```python
from build123d import *

# Parameters (mm, degrees)
BOSS_EXTRUDE1_DEPTH = 1.5875
FILLET1_R           = 2.54


with BuildPart() as part:
    # Sketch1 → Boss-Extrude1 (new body)
    with BuildSketch(Plane.XY):
        with BuildLine():
            Line((-5.175, 2.670071332), (-5.175, -5.175))
            Line((-5.175, -5.175), (5.175, -5.175))
            Line((5.175, -5.175), (5.175, 2.670071332))
            ThreePointArc((5.175, 2.670071332), (0, 12.7), (-5.175, 2.670071332))
        make_face()
        Polygon((-3.175, -1.5875), (-3.175, 1.5875), (-1.5875, 1.5875), (-1.5875, 3.175), (1.5875, 3.175), (1.5875, 1.5875), (3.175, 1.5875), (3.175, -1.5875), (1.5875, -1.5875), (1.5875, -3.175), (-1.5875, -3.175), (-1.5875, -1.5875), align=None, mode=Mode.SUBTRACT)
    extrude(amount=BOSS_EXTRUDE1_DEPTH)

    # Fillet1
    fillet1_edges = [part.edges().sort_by_distance(p)[0] for p in [
        (5.175, -5.175, 0.79375),
        (-5.175, -5.175, 0.79375),
    ]]
    fillet(fillet1_edges, radius=FILLET1_R)


solid = part.part
```
Input: part model. Units: mm. Frame: model coordinates. A direction names the side the tool comes from. Round coordinates to 2 decimals unless told otherwise and drop trailing zeros. Loops run counter-clockwise (first coordinate to the right, second up) from the corner with the lowest first, then second, coordinate; pieces in that order, holes last. Notation, with made-up numbers: (-2, 35) -> (49, 35) arc R23 ccw to (49, 70) -> close; hole circle Ø2 at (55.5, 84.25). An arc over 180 degrees is marked (long way). One line per item, written item: value.
(1) Section A-A (x = 0). Return the cut outline in (y, z) (1 decimal), plus the area to 3 significant figures.
Geometry check:
outline: (-5.2, 0) -> (-3.2, 0) -> (-3.2, 1.6) -> (-5.2, 1.6) -> close; (3.2, 0) -> (12.7, 0) -> (12.7, 1.6) -> (3.2, 1.6) -> close
area: 18.3 mm2
(2) Pin query (flat end, axial travel): pin 1 (0.5 mm diameter, centred on y = -0.5, z = 1, fed in from -X) (3 decimals); pin 2 (0.8 mm diameter, centred on x = -2, z = 1, fed in from +Y); pin 3 (3 mm diameter, centred on x = -1, y = 6.5, fed in from -Z); pin 4 (0.8 mm diameter, centred on y = 0.5, z = 1, fed in from +X) (3 decimals). Return the tip coordinate at first contact, or that it passes through.
Geometry check:
pin 1: x = -5.175
pin 2: y = 12.5
pin 3: z = 0
pin 4: x = 5.175
(3) Material intervals for line 1 (X direction, y = -0.25, z = 0.4) (3 decimals); line 2 (X direction, y = 2.5, z = 0.4) (1 decimal); line 3 (Y direction, x = -0.75, z = 0.35) (3 decimals), sorted ascending. Write a range as [from, to].
Geometry check:
line 1: [-5.175, -3.175], [3.175, 5.175]
line 2: [-5.2, -1.6], [1.6, 5.2]
line 3: [-5.175, -3.175], [3.175, 12.656]
(4) Set-up query: faces 1 (the face through (-5.175, 0, 1)), 2 (the face through (0, -5.175, 1)), 3 (the face through (0, -3.175, 1)). Return all of +Z, -Z, +X, -X, +Y, -Y with unobstructed straight access to the full face (end or side cutting, diameter ignored); none if empty.
Geometry check:
face 1: +Z, -Z, -X, -Y
face 2: +Z, -Z, +X, -X, -Y
face 3: +Z, -Z
(5) Mould query, pull axis Y, two halves, no side actions, for faces 4 (the face through (2, -1.588, 1)), 5 (the face through (0.195, 12.697, 0.783)), 6 (the face through (5.175, 0, 1)). Classes: pulls with the +Y half, pulls with the -Y half, needs draft (parallel to the pull), parting line crosses it, or undercut.
Geometry check:
face 4: undercut
face 5: parting line crosses it
face 6: needs draft
(6) Section C-C (x = -4). Return the cut outline in (y, z).
Geometry check:
outline: (-4.78, 0) -> (11.28, 0) -> (11.28, 1.59) -> (-4.78, 1.59) -> close
(7) Section D-D (y = 8.5). Return the cut outline in (x, z).
Geometry check:
outline: (-5.97, 0) -> (5.97, 0) -> (5.97, 1.59) -> (-5.97, 1.59) -> close
